```python
from build123d import *

# Parameters (mm, degrees)
SKETCH1_W           = 528.5
SKETCH1_H           = 43
SKETCH1_R           = 1.6
BOSS_EXTRUDE1_DEPTH = 4.5
SKETCH2_R           = 1.6
SKETCH2_W           = 15
SKETCH2_H           = 15
CUT_EXTRUDE1_DEPTH  = 5.5
FILLET1_R           = 3


with BuildPart() as part:
    # Sketch1 → Boss-Extrude1 (new body)
    with BuildSketch(Plane(origin=(0, 0, 0), x_dir=(1, 0, 0), z_dir=(0, 1, 0))):
        Rectangle(SKETCH1_W, SKETCH1_H)
        with Locations((-209.75, 10)):
            Circle(SKETCH1_R, mode=Mode.SUBTRACT)
        with Locations((-169.75, 10)):
            Circle(SKETCH1_R, mode=Mode.SUBTRACT)
        with Locations((-129.75, 10)):
            Circle(SKETCH1_R, mode=Mode.SUBTRACT)
        with Locations((-89.75, 10)):
            Circle(SKETCH1_R, mode=Mode.SUBTRACT)
        with Locations((-49.75, 10)):
            Circle(SKETCH1_R, mode=Mode.SUBTRACT)
        with Locations((-169.75, -10)):
            Circle(SKETCH1_R, mode=Mode.SUBTRACT)
        with Locations((-129.75, -10)):
            Circle(SKETCH1_R, mode=Mode.SUBTRACT)
        with Locations((-89.75, -10)):
            Circle(SKETCH1_R, mode=Mode.SUBTRACT)
        with Locations((-49.75, -10)):
            Circle(SKETCH1_R, mode=Mode.SUBTRACT)
        with Locations((-209.75, -10)):
            Circle(SKETCH1_R, mode=Mode.SUBTRACT)
        with Locations((234.25, 10)):
            Circle(SKETCH1_R, mode=Mode.SUBTRACT)
        with Locations((114.25, 10)):
            Circle(SKETCH1_R, mode=Mode.SUBTRACT)
        with Locations((114.25, -10)):
            Circle(SKETCH1_R, mode=Mode.SUBTRACT)
        with Locations((234.25, -10)):
            Circle(SKETCH1_R, mode=Mode.SUBTRACT)
        with Locations((134.25, -10)):
            Circle(SKETCH1_R, mode=Mode.SUBTRACT)
        with Locations((134.25, 10)):
            Circle(SKETCH1_R, mode=Mode.SUBTRACT)
        with Locations((254.25, 10)):
            Circle(SKETCH1_R, mode=Mode.SUBTRACT)
        with Locations((254.25, -10)):
            Circle(SKETCH1_R, mode=Mode.SUBTRACT)
        with Locations((94.25, -10)):
            Circle(SKETCH1_R, mode=Mode.SUBTRACT)
        with Locations((94.25, 10)):
            Circle(SKETCH1_R, mode=Mode.SUBTRACT)
        with Locations((214.25, 10)):
            Circle(SKETCH1_R, mode=Mode.SUBTRACT)
        with Locations((214.25, -10)):
            Circle(SKETCH1_R, mode=Mode.SUBTRACT)
    extrude(amount=BOSS_EXTRUDE1_DEPTH)

    # Sketch2 → Cut-Extrude1 (cut, through all)
    with BuildSketch(Plane(origin=(0, 4.5, 0), x_dir=(1, 0, 0), z_dir=(0, 1, 0))):
        with Locations((-256.75, 11.5)):
            Circle(SKETCH2_R)
        with Locations((-256.75, -11.5)):
            Circle(SKETCH2_R)
        with Locations((-256.75, 0)):
            Rectangle(SKETCH2_W, SKETCH2_H)
    extrude(amount=-CUT_EXTRUDE1_DEPTH, mode=Mode.SUBTRACT)

    # Fillet1
    fillet1_edges = [part.edges().sort_by_distance(p)[0] for p in [
        (-264.25, 2.25, 21.5),
        (-264.25, 2.25, -21.5),
    ]]
    fillet(fillet1_edges, radius=FILLET1_R)


solid = part.part
```
Can you work these out from the model? Positions are in its coordinate system, mm. Coordinates: 2 decimals unless noted, no trailing zeros. Answer as CSV lines item,"result". Start each with the question number.
1) Suppose I cut it at A-A (y = 3.1). Count the separate pieces of the cut face and the enclosed holes in it, plus the area to 3 significant figures.
2) For pin 1 (1.5 mm diameter, centred on y = 3.5, z = 4, fed in from -X); pin 2 (2.5 mm diameter, centred on x = 94.25, z = 10, fed in from +Y), each with a flat end and sliding along its axis, tell me the tip position at first contact or that it passes through.
3) I need wall thicknesses on line 1 (Z direction, x = 114.25, y = 2.2); line 2 (Z direction, x = 113.5, y = 4); line 3 (X direction, y = 3.25, z = 5.5). Which ranges of each line are inside material? Lowest first, please. Write a range as from..to.
Check result:
1,separate pieces,"1"
1,enclosed holes,"24"
1,area,"22,300 mm²"
2,pin 1,"stops at x = -249.25"
2,pin 2,"passes through"
3,line 1,"z = -21.5..-11.6, -8.4..8.4, 11.6..21.5"
3,line 2,"z = -21.5..-11.41, -8.59..8.59, 11.41..21.5"
3,line 3,"x = -249.25..264.25"
